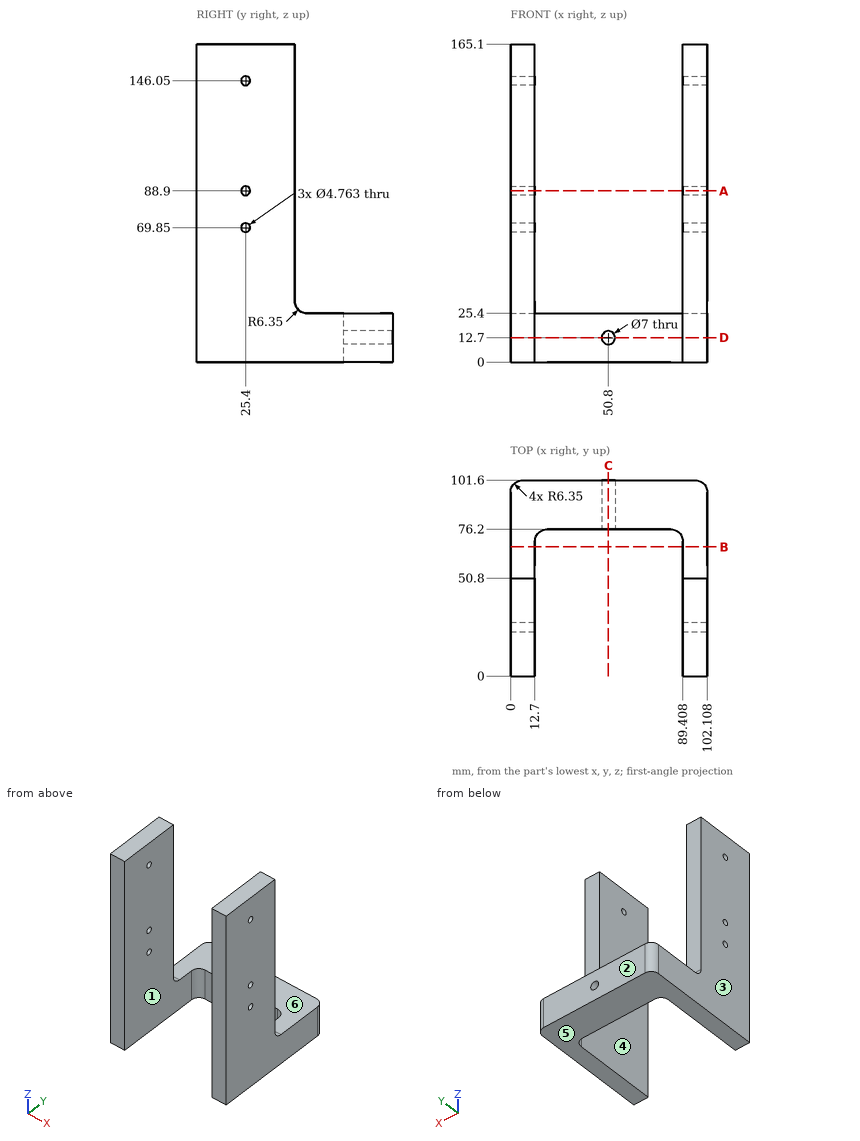
Here's the drawing with two shaded views (mm, measured from the low corner). I have some questions. A direction names the side the tool comes from. Coordinates: 2 decimals unless noted, no trailing zeros. Write each loop counter-clockwise with the first axis right and the second up, starting at its lowest first coordinate (ties: lowest second). Pieces come first, ordered by that corner, then holes. Notation, with made-up numbers: M -13,-16 L -3,-16 A10 ccw -3,-9 Z; hole C 33.25,87 d4. An arc over 180 degrees is marked long. Write item = value, one per line. Start each with the question number.
Q1. If we section it at A-A, the plane z = 88.9: Write out the boundary of the cut face in (x, y), then the cut area to 3 significant figures.
Q2. If we section it at D-D, the plane z = 12.7: Write out the boundary of the cut face in (x, y).
Q3. I'm going to push flat-ended pins straight in: pin 1 (14 mm diameter, centred on x = 96.5, z = 91, fed in from +Y); pin 2 (12.5 mm diameter, centred on x = 57.5, z = 9, fed in from -Y). Where does each tip first touch, or does it pass through?
Q4. Thinking about a two-plate mould opening in X: for the marked faces 1, 2 and 3, which applies, released by +X, released by -X, zero draft, split by the parting line, or undercut?
Q5. If we section it at C-C, the plane x = 50.8: Write out the boundary of the cut face in (y, z), then the cut area to 3 significant figures.
Q6. On a 3-axis mill with a long thin cutter (end or side, diameter ignored), from which of +Z, -Z, +X, -X, +Y, -Y can I reach the whole of each face in a straight line? I mean the marked faces 4, 5 and 6. Say none if no direction works.
Q7. If we section it at B-B, the plane y = 67: Write out the boundary of the cut face in (x, z), then the cut area to 3 significant figures.
Q8. If I drill on L1, parallel to Z at x = 6, y = 25; L2, parallel to X at y = 40.5, z = 76.5; L3, parallel to Y at x = 10, z = 146, over which ranges is the centre line in solid material (lowest first)? Write a range as [from, to].
Check sheet entries:
q1.outline = M 0,0 L 12.7,0 L 12.7,23.02 L 0,23.02 Z; M 0,27.78 L 12.7,27.78 L 12.7,50.8 L 0,50.8 Z; M 89.41,0 L 102.11,0 L 102.11,23.02 L 89.41,23.02 Z; M 89.41,27.78 L 102.11,27.78 L 102.11,50.8 L 89.41,50.8 Z
q1.area = 1,170 mm²
q2.outline = M 0,0 L 12.7,0 L 12.7,69.85 A6.35 cw 19.05,76.2 L 47.3,76.2 L 47.3,101.6 L 6.35,101.6 A6.35 ccw 0,95.25 Z; M 54.3,76.2 L 83.06,76.2 A6.35 cw 89.41,69.85 L 89.41,0 L 102.11,0 L 102.11,95.25 A6.35 ccw 95.76,101.6 L 54.3,101.6 Z
q3.pin_1 = 50.8
q3.pin_2 = 76.2
q4.face_1 = undercut
q4.face_2 = zero draft
q4.face_3 = released by -X
q5.outline = M 76.2,0 L 101.6,0 L 101.6,9.2 L 76.2,9.2 Z; M 76.2,16.2 L 101.6,16.2 L 101.6,25.4 L 76.2,25.4 Z
q5.area = 467 mm²
q6.face_4 = +Z, -Z, -Y
q6.face_5 = -Z, +X, -X, +Y, -Y
q6.face_6 = +Z, +X, -X, +Y
q7.outline = M 0,0 L 12.7,0 L 12.7,25.4 L 0,25.4 Z; M 89.41,0 L 102.11,0 L 102.11,25.4 L 89.41,25.4 Z
q7.area = 645 mm²
q8.L1 = [0, 67.5], [72.2, 86.55], [91.25, 143.7], [148.4, 165.1]
q8.L2 = [0, 12.7], [89.41, 102.11]
q8.L3 = [0, 23.02], [27.78, 50.8]
